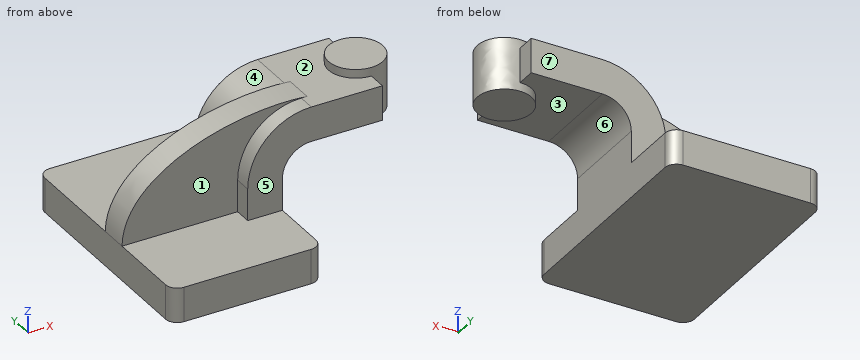
```python
from build123d import *

# Parameters (mm, degrees)
F1_DEPTH = 63.5
F2_DEPTH = 25.4
F3_DEPTH = 15.875
F5_R     = 6.35


with BuildPart() as f1:
    # F0 (on Front) → F1 (new body, symmetric)
    with BuildSketch(Plane.XZ):
        Polygon((41.275, -9.525), (41.275, 9.525), (22.225, 9.525), (-41.275, 9.525), (-41.275, -9.525), align=None)
    extrude(amount=F1_DEPTH, both=True)

    # F0 (on Front) → F2 (join, symmetric)
    with BuildSketch(Plane.XZ):
        with BuildLine():
            Line((22.225, 9.525), (41.275, 9.525))
            Line((41.275, 9.525), (41.275, 27.0002))
            ThreePointArc((41.275, 27.0002), (45.9246798487, 38.2255201513), (57.15, 42.8752))
            Line((57.15, 42.8752), (60.325, 42.8752))
            Line((60.325, 42.8752), (60.325, 61.9252))
            Line((60.325, 61.9252), (57.15, 61.9252))
            ThreePointArc((57.15, 61.9252), (32.4542956671, 51.6959043329), (22.225, 27.0002))
            Line((22.225, 27.0002), (22.225, 9.525))
        make_face()
        Polygon((96.2208863549, 61.9252), (60.325, 61.9252), (60.325, 42.8752), (96.2274231248, 42.8752), align=None)
    extrude(amount=F2_DEPTH, both=True)

    # F0 (on Front) → F3 (join)
    with BuildSketch(Plane.XZ):
        with BuildLine():
            Line((-41.275, 9.525), (22.225, 9.525))
            Line((22.225, 9.525), (22.225, 27.0002))
            ThreePointArc((22.225, 27.0002), (32.4542956671, 51.6959043329), (57.15, 61.9252))
            Line((57.15, 61.9252), (60.325, 61.9252))
            add(Edge.make_bspline(
                [(-41.275, 9.525), (-40.5514836311, 47.1779592335), (18.5578372329, 65.8548623323), (60.325, 61.9252)],
                knots=[0, 0, 0, 0, 114.3168446032, 114.3168446032, 114.3168446032, 114.3168446032], degree=3))
        make_face()
    extrude(amount=F3_DEPTH)

    # F0 (on Front) → F4 (revolve)
    with BuildSketch(Plane.XZ):
        Polygon((96.2192565203, 66.675), (96.2208863549, 61.9252), (96.2274231248, 42.8752), (96.2290616752, 38.1), (111.125, 38.1), (111.125, 66.675), align=None)
    revolve(axis=Axis((96.2241590977, 0, 52.3875), (0.0003431375, 0, -0.9999999411)))

    # F5
    f5_edges = [f1.edges().sort_by_distance(p)[0] for p in [
        (41.275, -63.5, 0),
        (-41.275, -63.5, 0),
        (-41.275, 63.5, 0),
        (41.275, 63.5, 0),
    ]]
    fillet(f5_edges, radius=F5_R)


solid = f1.part
```
Design review of the part built by this model. Coordinates are the model's own, in mm. Face numbers are marked on the shaded views. A direction names the side the tool comes from. Give positions to 0.01 mm unless a question says otherwise; leave off trailing zeros. Order: outer loops, then holes, each group sorted by start corner. A loop starts at its lowest first (then second) coordinate and runs counter-clockwise, first axis right, second up. Notation, with made-up numbers: (64.25, 14) - (83.25, 14) arc R12 ccw to (83.25, 25) - close; hole circle Ø7 at (-31.75, 50). An arc over 180 degrees is marked (long way). Use a Markdown table: item, result. Add a question column.
(1) Add section A-A on z = 6.5. Give the boundary of the cut face in (x, y) (3 decimals), then the cut area to 3 significant figures.
(2) Add section C-C on y = 34. Give the boundary of the cut face in (x, z) (3 decimals).
(3) Clearance check with flat-ended pins moving along their axes: P1, Ø8.5, axis at y = 17.5, z = 55, coming from the +X side; P2, Ø2, axis at y = -10, z = 42, coming from the -X side; P3, Ø5, axis at x = 83.5, y = -13, coming from the -Z side. State where each tip first meets the part, or that it passes through.
(4) Mouldability with a two-part tool opening along X and no side actions: class the marked faces 1, 2, 3 and 4 as +X half, -X half, draft (parallel to the pull), parting line (faces both ways), or undercut.
(5) Add section B-B on x = 62.5. Give the boundary of the cut face in (y, z).
(6) Wall thickness on probe 1 along Z at (x, y) = (31, -57.5) (3 decimals); probe 2 along X at (y, z) = (2, 23.5) (3 decimals); probe 3 along Y at (x, z) = (-21.5, 22) (3 decimals): over which ranges is each line inside the solid? List them lowest first. Write a range as [from, to].
(7) Machinability: for the marked faces 5, 6 and 7, which of the approach directions +Z, -Z, +X, -X, +Y, -Y give a long, thin tool a straight path to every point of the face, cutting with its end or side? Answer none if there is none.
Report:
| question | item | result |
|---|---|---|
| 1 | outline | (-41.275, -57.15) arc R6.35 ccw to (-34.925, -63.5) - (34.925, -63.5) arc R6.35 ccw to (41.275, -57.15) - (41.275, 57.15) arc R6.35 ccw to (34.925, 63.5) - (-34.925, 63.5) arc R6.35 ccw to (-41.275, 57.15) - close |
| 1 | area | 10,400 mm² |
| 2 | outline | (-41.275, -9.525) - (41.275, -9.525) - (41.275, 9.525) - (-41.275, 9.525) - close |
| 3 | P1 | stops at x = 103.04 |
| 3 | P2 | stops at x = -23.53 |
| 3 | P3 | stops at z = 42.88 |
| 4 | face 1 | draft |
| 4 | face 2 | undercut |
| 4 | face 3 | undercut |
| 4 | face 4 | -X half |
| 5 | outline | (-25.4, 42.88) - (25.4, 42.88) - (25.4, 61.93) - (-25.4, 61.93) - close |
| 6 | probe 1 | z = [-9.525, 9.525] |
| 6 | probe 2 | x = [22.225, 41.275] |
| 6 | probe 3 | y = [-15.875, 0] |
| 7 | face 5 | +Z, +X, -X, -Y |
| 7 | face 6 | -Z, +Y, -Y |
| 7 | face 7 | +Z, +X, -X, +Y |
